Check sheet for the modelled part. Datum: model origin and axes. Units: mm. Face numbers are marked on the shaded views. A direction names the side the tool comes from. Coordinates: 2 decimals unless noted, no trailing zeros. Loops run counter-clockwise (first coordinate to the right, second up) from the corner with the lowest first, then second, coordinate; pieces in that order, holes last. Notation, with made-up numbers: M -3.5,66.25 L 42.5,66.25 A31 ccw 42.5,100.25 Z; hole C -27.75,58.25 d9. An arc over 180 degrees is marked long. Use CSV: the item, a comma, the result in double quotes. Start each with the question number.
(1) Draft check along Y on the marked faces 3, 4, 5 and 6. Enter one of: pulls with the +Y half, pulls with the -Y half, needs draft (parallel to the pull), parting line crosses it, or undercut.
(2) Scan lines: line 1 (Y direction, x = -0.25, z = 0) (3 decimals); line 2 (Z direction, x = -5, y = -1); line 3 (Y direction, x = -36, z = -41.5) (3 decimals). Record each from-to range of solid material in increasing order.
(3) Set-up check for the marked faces 1 and 2: record each of +Z, -Z, +X, -X, +Y, -Y from which the full face is reachable in a straight line by a thin tool's end or side.
(4) Section check A-A on y = 4. Record the cut outline in (x, z).
(5) Go/stop test with flat-tipped pins: pin 1 Ø2.5 at (y, z) = (7.59, 0) entering from +X; pin 2 Ø8 at (y, z) = (6.5, -39) entering from +X; pin 3 Ø3 at (y, z) = (8, -44.5) entering from -X. Record where each tip stops, or that it passes through.
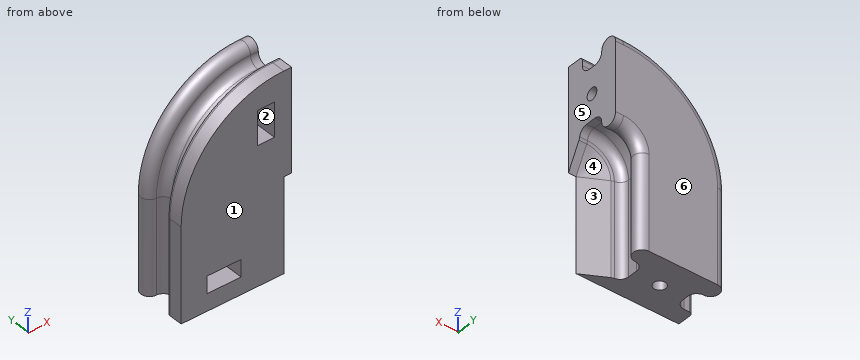
Autodesk Inventor part; units mm, degrees
ref_plane "YZ Plane" through (0, 0, 0) normal (1, 0, 0) x (0, 1, 0)
ref_plane "XZ Plane" through (0, 0, 0) normal (0, 1, 0) x (-1, 0, 0)
ref_plane "XY Plane" through (0, 0, 0) normal (0, 0, 1) x (1, 0, 0)
sketch "Sketch1" plane through (0, 0, 0) normal (1, 0, 0) x (0, 1, 0)
  line L0 (-3.175, -15.8752) -> (-3.175, 15.8752)
  line L1 (-3.175, 15.8752) -> (1.9596, -9.7981) construction
  line L2 (3.175, 15.8752) -> (-3.175, -15.8752) construction
  arc A0 (18.3756, 12.7) -> (12.0256, 12.7001) centre (15.2006, 12.7) ccw
  arc A1 (12.0256, -12.7001) -> (18.3756, -12.7) centre (15.2006, -12.7) ccw
  line L3 (8.8506, 9.5252) -> (6.35, 9.5252)
  line L4 (8.8506, -9.5252) -> (5.1346, -9.5252)
  line L5 (15.2006, 12.7) -> (15.2006, -12.7) construction
  line L6 (3.175, 14.6052) -> (3.175, 12.7002)
  arc A2 (8.8506, 9.5252) -> (12.0256, 12.7001) centre (8.8506, 12.7002) ccw
  arc A3 (12.0256, -12.7001) -> (8.8506, -9.5252) centre (8.8506, -12.7002) ccw
  arc A4 (3.175, 12.7002) -> (6.35, 9.5252) centre (6.35, 12.7002) ccw
  arc A5 (5.1346, -9.5252) -> (1.9937, -12.2364) centre (5.1346, -12.7002) ccw
  line L7 (-3.175, -15.8752) -> (-3.175, -22.2252)
  line L8 (1.905, 15.8752) -> (-3.175, 15.8752)
  arc A6 (3.175, 14.6052) -> (1.905, 15.8752) centre (1.905, 14.6052) ccw
  line L9 (18.3756, 12.7) -> (18.3756, -12.7)
  line L10 (1.6475, -13.2791) -> (-3.175, -22.2252)
  arc A7 (1.6475, -13.2791) -> (1.9937, -12.2364) centre (-1.1473, -11.7726) ccw
  line L11 (-3.175, -22.2252) -> (20.4919, -22.2252)
  point P0 (0, 0)
  point P1 (15.2367, 9.5252)
  point P2 (15.2367, -9.5252)
  point P3 (1.9596, -12.7002)
  dimension "d5" = 6.35
  dimension "d8" = 3.175
  dimension "d9" = 6.35
  dimension "d11" = 6.35
  dimension "d12" = 6.35
  dimension "d13" = 1.27
  dimension "d30" = 25.4
  dimension "d31" = 3.175
revolve "Revolution1" add sketch "Sketch1" angle 90 about axis through (0, -3.175, -22.2252) along (0, -1, 0)
extrude "Extrusion2" add sketch "Sketch1" along normal blind 2.8575
sketch "Sketch2" plane through (-9.5252, 18.3756, -22.2252) normal (0, 0, -1) x (-1, 0, 0)
  line L0 (-9.5252, -21.5506) -> (28.5752, -21.5506)
  line L1 (28.5752, -21.5506) -> (28.5752, -16.4706)
  arc A0 (28.5752, -16.4706) -> (27.3052, -15.2006) centre (27.3052, -16.4706) ccw
  line L2 (27.3052, -15.2006) -> (25.4002, -15.2006)
  arc A1 (22.2252, -12.0256) -> (25.4002, -15.2006) centre (25.4002, -12.0256) ccw
  line L3 (22.2252, -12.0256) -> (22.2252, -9.525)
  arc A2 (25.4001, -6.35) -> (22.2252, -9.525) centre (25.4002, -9.525) ccw
  arc A3 (25.4001, -6.35) -> (25.4, 0) centre (25.4, -3.175) ccw
  line L4 (25.4, 0) -> (0, 0)
  arc A4 (0, 0) -> (-0.0001, -6.35) centre (0, -3.175) ccw
  arc A5 (3.1748, -9.525) -> (-0.0001, -6.35) centre (-0.0002, -9.525) ccw
  line L5 (3.1748, -9.525) -> (3.1748, -13.241)
  arc A6 (0.4636, -16.382) -> (3.1748, -13.241) centre (-0.0002, -13.241) ccw
  arc A7 (0.4636, -16.382) -> (-0.5791, -16.7281) centre (0.9274, -19.5229) ccw
  line L6 (-0.5791, -16.7281) -> (-9.5252, -21.5506)
  point P0 (-9.5252, -18.3756)
extrude "Extrusion3" add sketch "Sketch2" along normal blind 34.925
sketch "Sketch5" plane through (2.8575, 0, 0) normal (1, 0, 0) x (0, 0, -1)
  circle A0 centre (0, 7.5946) radius 2.2225
  line L0 (-15.8752, -3.175) -> (22.2252, -3.175)
  point P0 (0, 0)
  dimension "d26" = 4.445
  dimension "d27" = 10.7696
extrude "Extrusion4" cut sketch "Sketch5" against normal blind 12.7
sketch "Sketch6" plane through (-9.5252, 18.3756, -57.1502) normal (0, 0, -1) x (-1, 0, 0)
  line L0 (3.1748, -9.525) -> (3.1748, -13.241)
  line L1 (3.1748, -10.781) -> (22.2252, -10.781) construction
  line L2 (22.2252, -12.0256) -> (22.2252, -9.525)
  circle A0 centre (12.7, -10.781) radius 2.2225
  line L3 (-9.5252, -21.5506) -> (28.5752, -21.5506)
  point P0 (-9.5252, -18.3756)
  dimension "d32" = 4.445
  dimension "d33" = 10.7696
extrude "Extrusion5" cut sketch "Sketch6" against normal blind 12.7
sketch "Sketch7" plane through (0, -3.175, 15.8752) normal (0, -1, 0) x (1, 0, 0)
  line L0 (-9.8425, -13.6527) -> (-9.8425, -18.0977)
  line L1 (2.8575, -13.6527) -> (2.8575, -18.0977)
  line L2 (-20.0027, -60.3254) -> (-24.4477, -60.3254)
  line L3 (-20.0027, -73.0254) -> (-24.4477, -73.0254)
  line L4 (2.8575, 0) -> (2.8575, -38.1004)
  line L5 (2.8575, -15.8752) -> (-3.4925, -15.8752) construction
  line L6 (-9.8425, -22.2252) -> (-3.4925, -22.2252)
  line L7 (-3.4925, -22.2252) -> (-3.4925, -9.5252)
  line L8 (-3.4925, -9.5252) -> (-9.8425, -9.5252)
  line L9 (-9.8425, -9.5252) -> (-9.8425, -22.2252)
  line L10 (-9.8425, -22.2252) -> (-3.4925, -9.5252) construction
  line L11 (-3.4925, -22.2252) -> (-9.8425, -9.5252) construction
  line L12 (0, -73.0254) -> (-38.1004, -73.0254)
  line L13 (-22.2252, -73.0254) -> (-22.2252, -66.6754) construction
  line L14 (-15.8752, -60.3254) -> (-28.5752, -60.3254)
  line L15 (-28.5752, -60.3254) -> (-28.5752, -66.6754)
  line L16 (-28.5752, -66.6754) -> (-15.8752, -66.6754)
  line L17 (-15.8752, -66.6754) -> (-15.8752, -60.3254)
  line L18 (-15.8752, -60.3254) -> (-28.5752, -66.6754) construction
  line L19 (-28.5752, -60.3254) -> (-15.8752, -66.6754) construction
  point P0 (0, -15.8752)
  point P1 (-6.6675, -15.8752)
  point P2 (-22.2252, -63.5004)
  dimension "d41" = 6.35
  dimension "d42" = 6.35
  dimension "d43" = 12.7
  dimension "d44" = 6.35
extrude "Extrusion6" cut sketch "Sketch7" against normal blind 17.145
fillet "Fillet1" radius 6.35 4 edges at (-6.6675, 13.97, 6.35) (-6.6675, 13.97, -6.35) (-28.5752, 13.97, -47.6252) (-15.8752, 13.97, -47.6252)
properties part number "Rail Corner 2" material "Acetal Resin, Black"
Outcome:
1,face 3,"undercut"
1,face 4,"undercut"
1,face 5,"needs draft"
1,face 6,"pulls with the +Y half"
2,line 1,"y = -3.175 to 5.372, 9.817 to 18.376"
2,line 2,"z = -57.15 to -6.35, 6.35 to 15.55"
2,line 3,"y = -3.175 to 3.175, 12.213 to 18.188"
3,face 1,"+Z, -Z, +X, -X, -Y"
3,face 2,"-Y"
4,outline,"M -32.79,-57.15 L -12.49,-57.15 L -12.49,-22.23 A12.49 cw 0,-9.73 L 2.86,-9.73 L 2.86,10.57 L 0,10.57 A32.79 ccw -32.79,-22.23 Z; hole M -28.58,-50.8 L -15.88,-50.8 L -15.88,-44.45 L -28.58,-44.45 Z; hole M -9.84,-6.35 L -3.49,-6.35 L -3.49,6.35 L -9.84,6.35 Z"
5,pin 1,"stops at x = -9.84"
5,pin 2,"stops at x = -11.3"
5,pin 3,"stops at x = -31.82"
